Part model, mm, in its own coordinate system. Face numbers are marked on the shaded views. A direction names the side the tool comes from. Round coordinates to 2 decimals unless told otherwise and drop trailing zeros. Write each loop counter-clockwise with the first axis right and the second up, starting at its lowest first coordinate (ties: lowest second). Pieces come first, ordered by that corner, then holes. Notation, with made-up numbers: (-22, 60.5) -> (-13, 60.5) arc R20 cw to (-13, 78.5) -> close; hole circle Ø10 at (11, -35.5). An arc over 180 degrees is marked (long way). Return JSON: item names as keys, results as strings. Group by question number.
```python
from build123d import *

# Parameters (mm, degrees)
F0_W      = 108
F0_H      = 24
F1_DEPTH  = 72
F3_DEPTH  = 6
F4_DEPTH  = 24.001
F6_DEPTH  = 6
F8_DEPTH  = 30.001
F9_R      = 9
F10_DEPTH = 3
F11_DEPTH = 24.001


with BuildPart() as f1:
    # F0 (on Front) → F1 (new body)
    with BuildSketch(Plane.XZ):
        with Locations((3.6308863163, -7.8423750699)):
            Rectangle(F0_W, F0_H)
    extrude(amount=F1_DEPTH)

    # F2 (on face) → F3 (cut)
    with BuildSketch(Plane.XY.offset(4.1576249301)):
        with BuildLine():
            Line((-50.3691136837, -48), (-50.3691136837, -60))
            Line((-50.3691136837, -60), (-38.3691136837, -60))
            ThreePointArc((-38.3691136837, -60), (-14.3691136837, -36), (-38.3691136837, -12))
            Line((-38.3691136837, -12), (-50.3691136837, -12))
            Line((-50.3691136837, -12), (-50.3691136837, -24))
            Line((-50.3691136837, -24), (-38.3691136837, -24))
            ThreePointArc((-38.3691136837, -24), (-26.3691136837, -36), (-38.3691136837, -48))
            Line((-38.3691136837, -48), (-50.3691136837, -48))
        make_face()
    extrude(amount=-F3_DEPTH, mode=Mode.SUBTRACT)

    # F4 (cut, through all): a face of the model
    f4_faces = [f1.faces().sort_by_distance(p)[0] for p in [
        (-39.4893119907, -36, 4.1576249301),
    ]]
    extrude(f4_faces, amount=-F4_DEPTH, mode=Mode.SUBTRACT)

    # F5 (on face) → F6 (join)
    with BuildSketch(Plane.XY.offset(4.1576249301)):
        Polygon((21.6308863163, 0), (-14.3691136837, 0), (-14.3691136837, -36), (-14.3691136837, -54), (21.6308863163, -54), align=None)
    extrude(amount=F6_DEPTH)

    # F7 (on face) → F8 (cut, through all)
    with BuildSketch(Plane.XY.offset(10.1576249301)):
        with BuildLine():
            ThreePointArc((3.6308863163, -12), (-0.6117543708, -22.2426406871), (9.6308863163, -18))
            ThreePointArc((9.6308863163, -18), (7.8735270034, -13.7573593129), (3.6308863163, -12))
        make_face()
    extrude(amount=-F8_DEPTH, mode=Mode.SUBTRACT)

    # F9 (on face) → F10 (join)
    with BuildSketch(Plane.XY.offset(4.1576249301)):
        with BuildLine():
            Line((21.6308863163, -54), (39.6308863163, -54))
            ThreePointArc((39.6308863163, -54), (57.6308863163, -36), (39.6308863163, -18))
            Line((39.6308863163, -18), (21.6308863163, -18))
            Line((21.6308863163, -18), (21.6308863163, -54))
        make_face()
        with Locations((39.6308863163, -36)):
            Circle(F9_R, mode=Mode.SUBTRACT)
    extrude(amount=F10_DEPTH)

    # F11 (cut, through all): a face of the model
    f11_faces = [f1.faces().sort_by_distance(p)[0] for p in [
        (39.6308863163, -36, 4.1576249301),
    ]]
    extrude(f11_faces, amount=-F11_DEPTH, mode=Mode.SUBTRACT)


solid = f1.part
```
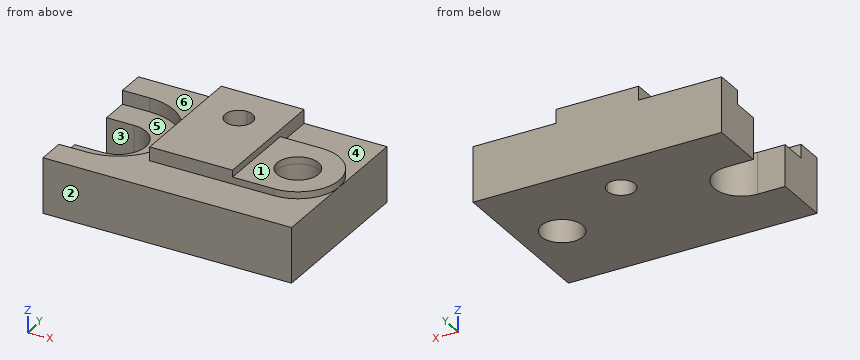
Item 1: Cut at C-C (y = -33.5). Write the cut outline in (x, z), then the cut area to 3 significant figures.
Item 2: Cut at A-A (z = -12). Write the cut outline in (x, y), then the cut area to 3 significant figures.
Item 3: Cut at B-B (x = -44). Write the cut outline in (y, z).
Item 4: Flat gauge pins, fed straight in: P1, Ø3.5, axis at x = 30.5, z = 6, coming from the +Y side; P2, Ø5, axis at x = 3, z = 7.5, coming from the -Y side; P3, Ø10, axis at x = 29.5, z = -6, coming from the +Y side; P4, Ø18, axis at x = -26.5, y = -42.5, coming from the +Z side. Where does each tip first touch, or does it go through?
Item 5: Wall check: L1, parallel to Y at x = -39, z = -3; L2, parallel to Z at x = -17, y = -66; L3, parallel to Z at x = 28, y = -42. Give the ranges that are in metal, low to high.
Item 6: Cut at D-D (x = -19). Write the cut outline in (y, z).
Item 7: Which spindle directions (+Z, -Z, +X, -X, +Y, -Y) get a long thin tool onto all of the face, cutting with end or side? Do the marked faces 4, 5 and 6. Say none if no direction does.
Item 8: Two-plate mould, pull along Y, no slides. Class the marked faces 1, 2 and 3: released by +Y, released by -Y, zero draft, split by the parting line, or undercut.
Checks:
{
 "1": {"outline": "(-26.63, -19.84) -> (30.99, -19.84) -> (30.99, 7.16) -> (21.63, 7.16) -> (21.63, 10.16) -> (-14.37, 10.16) -> (-14.37, 4.16) -> (-14.5, 4.16) -> (-14.5, -1.84) -> (-26.63, -1.84) -> close; (48.28, -19.84) -> (57.63, -19.84) -> (57.63, 4.16) -> (57.46, 4.16) -> (57.46, 7.16) -> (48.28, 7.16) -> close", "area": "1,810 mm2"},
 "2": {"outline": "(-50.37, -72) -> (57.63, -72) -> (57.63, 0) -> (-50.37, 0) -> (-50.37, -24) -> (-38.37, -24) arc R12 cw to (-38.37, -48) -> (-50.37, -48) -> close; hole circle Ø12 at (3.63, -18); hole circle Ø18 at (39.63, -36)", "area": "6,890 mm2"},
 "3": {"outline": "(-72, -19.84) -> (-48, -19.84) -> (-48, -1.84) -> (-60, -1.84) -> (-60, 4.16) -> (-72, 4.16) -> close; (-24, -19.84) -> (0, -19.84) -> (0, 4.16) -> (-12, 4.16) -> (-12, -1.84) -> (-24, -1.84) -> close"},
 "4": {"P1": "stops at y = -18", "P2": "stops at y = -54", "P3": "stops at y = 0", "P4": "stops at z = -1.84"},
 "5": {"L1": "y = -72 to -48, -24 to 0", "L2": "z = -19.84 to 4.16", "L3": "z = -19.84 to 7.16"},
 "6": {"outline": "(-72, -19.84) -> (0, -19.84) -> (0, 4.16) -> (-21.83, 4.16) -> (-21.83, -1.84) -> (-50.17, -1.84) -> (-50.17, 4.16) -> (-72, 4.16) -> close"},
 "7": {"face 4": "+Z, +X, +Y", "face 5": "+Z, -X", "face 6": "+Z, -X, +Y, -Y"},
 "8": {"face 1": "zero draft", "face 2": "released by -Y", "face 3": "undercut"}
}
